Could you check a few things on this model? Use its own coordinates, in mm. Face numbers are marked on the shaded views. A direction names the side the tool comes from. Round coordinates to 2 decimals unless told otherwise and drop trailing zeros. Loops run counter-clockwise (first coordinate to the right, second up) from the corner with the lowest first, then second, coordinate; pieces in that order, holes last. Notation, with made-up numbers: M 61.25,79.5 L 75.25,79.5 A20 ccw 75.25,103.5 Z; hole C -5.5,84.5 d2. An arc over 180 degrees is marked long. Answer in a Markdown table with one row per item.
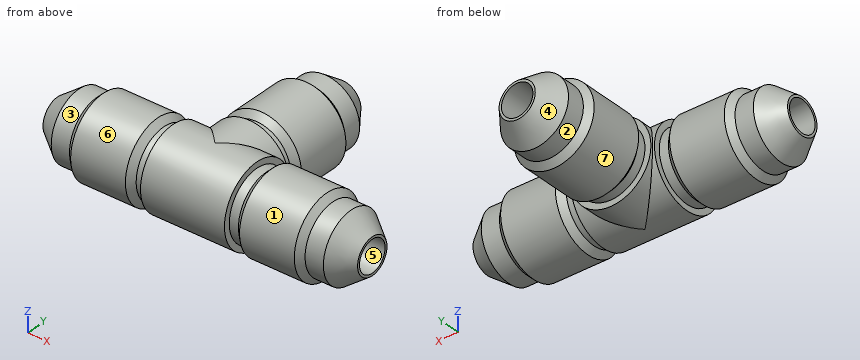
```python
from build123d import *

# Parameters (mm, degrees)
SKETCH2_R           = 5.55625
EXTRUDE1_DEPTH      = 16.002
SKETCH15_R          = 5.55625
BOSS_EXTRUDE1_DEPTH = 5.826125
SKETCH16_R          = 2.1844
CUT_EXTRUDE1_DEPTH  = 24.199372171
CIRPATTERN1_COUNT   = 3
CIRPATTERN1_ANGLE   = 180
SKETCH17_R          = 2.1844
CUT_EXTRUDE2_DEPTH  = 50.124404517
CUT_EXTRUDE3_REACH  = 37.458
SKETCH18_R          = 2.1844


with BuildPart() as part:
    # Sketch2 → Extrude1 (new body)
    with BuildSketch(Plane(origin=(-21.828125, 0, 0), x_dir=(0, 0, -1), z_dir=(1, 0, 0))):
        Circle(SKETCH2_R)
    extrude(amount=EXTRUDE1_DEPTH)

    # Sketch5 → Cut-Revolve1 (revolve, cut)
    with BuildSketch(Plane.XY, mode=Mode.PRIVATE) as cut_revolve1_sk:
        Polygon((-18.883013362, 4.731360803), (-16.343013362, 4.731360803), (-15.518124165, 5.55625), (-21.828125, 5.55625), (-21.828125, 2.51206), align=None)
        Polygon((-5.826125, 4.731360803), (-7.096125, 4.731360803), (-7.921014197, 5.55625), (-5.826125, 5.55625), align=None)
    revolve(cut_revolve1_sk.sketch.rotate(Axis((0, 0, 0), (-1, 0, 0)), 90), axis=Axis((0, 0, 0), (-1, 0, 0)), mode=Mode.SUBTRACT)

    # Sketch15 → Boss-Extrude1 (add)
    with BuildSketch(Plane(origin=(-5.826125, 0, 0), x_dir=(0, 0, -1), z_dir=(1, 0, 0))):
        Circle(SKETCH15_R)
    extrude(amount=BOSS_EXTRUDE1_DEPTH)

    # Sketch16 → Cut-Extrude1 (cut, through all)
    with BuildSketch(Plane(origin=(0, 0, 0), x_dir=(0, 0, -1), z_dir=(1, 0, 0))):
        Circle(SKETCH16_R)
    extrude(amount=-CUT_EXTRUDE1_DEPTH, mode=Mode.SUBTRACT)


with BuildPart() as cirpattern1_1:
    # CirPattern1: pattern copy
    add(part.part.rotate(Axis((0, 0, 0), (0, 0, -1)), 1 * CIRPATTERN1_ANGLE / (CIRPATTERN1_COUNT - 1)))

    # Sketch17 → Cut-Extrude2 (cut, through all)
    with BuildSketch(Plane.ZY.offset(21.828125)):
        with Locations(Location((0, 0, 0), (0, 0, 180))):
            Circle(SKETCH17_R)
    extrude(amount=-CUT_EXTRUDE2_DEPTH, mode=Mode.SUBTRACT)


with BuildPart() as cirpattern1_2:
    # CirPattern1: pattern copy
    add(part.part.rotate(Axis((0, 0, 0), (0, 0, -1)), 2 * CIRPATTERN1_ANGLE / (CIRPATTERN1_COUNT - 1)))


with BuildPart() as cirpattern1_1_1:
    add(cirpattern1_1.part)

    # Combine1: union part, CirPattern1_2
    add(part.part)
    add(cirpattern1_2.part)

    # Sketch18 → Cut-Extrude3 (cut, up to next)
    with BuildSketch(Plane(origin=(0, 21.828125, 0), x_dir=(1, 0, 0), z_dir=(0, 1, 0)), mode=Mode.PRIVATE) as cut_extrude3_sk1:
        with Locations(Location((0, 0, 0), (0, 0, 90))):
            Circle(SKETCH18_R)
    cut_extrude3_tool1 = extrude(cut_extrude3_sk1.sketch, amount=-CUT_EXTRUDE3_REACH, mode=Mode.PRIVATE) & cirpattern1_1_1.part
    add(cut_extrude3_tool1.solids().sort_by_distance((0, 21.828125, 0))[0], mode=Mode.SUBTRACT)


solid = cirpattern1_1_1.part
```
1) I want a section at B-B, the plane x = 0. Please give me the cut outline in (y, z), plus the area to 3 significant figures.
Computed:
| item | result |
|---|---|
| outline | M 0,-5.56 L 5.83,-5.56 L 5.83,-4.73 L 7.1,-4.73 L 7.92,-5.56 L 15.52,-5.56 L 16.34,-4.73 L 18.88,-4.73 L 21.83,-2.51 L 21.83,-2.18 L 0,-2.18 A2.18 cw 0,2.18 L 21.83,2.18 L 21.83,2.51 L 18.88,4.73 L 16.34,4.73 L 15.52,5.56 L 7.92,5.56 L 7.1,4.73 L 5.83,4.73 L 5.83,5.56 L 0,5.56 A5.56 ccw Z |
| area | 169 mm² |
2) I want a section at C-C, the plane z = 0. State how many separate pieces and enclosed holes the cut face has, plus the area to 3 significant figures.
Computed:
| item | result |
|---|---|
| separate pieces | 3 |
| enclosed holes | 0 |
| area | 332 mm² |
3) I need wall thicknesses on line 1 (X direction, y = 13.75, z = 0); line 2 (X direction, y = 17.5, z = 0); line 3 (Y direction, x = 0.5, z = 0). Which ranges of each line are inside material? Lowest first, please.
Computed:
| item | result |
|---|---|
| line 1 | x = -5.56 to -2.18, 2.18 to 5.56 |
| line 2 | x = -4.73 to -2.18, 2.18 to 4.73 |
| line 3 | y = -5.56 to -2.18 |
4) Will these pins go through, and if not, where does the flat tip stop? P1, Ø1.5, axis at x = -12, y = 5.5, coming from the -Z side; P2, Ø1, axis at x = -5, y = 10, coming from the -Z side; P3, Ø1, axis at x = -2, z = -4, coming from the +Y side.
Computed:
| item | result |
|---|---|
| P1 | stops at z = -2.88 |
| P2 | stops at z = -3.26 |
| P3 | stops at y = 19.89 |
5) If we mould it in two halves opening along Y, with no side actions, what happens to the marked faces 4, 5, 6 and 7? For each: released by +Y, released by -Y, zero draft, split by the parting line, or undercut.
Computed:
| item | result |
|---|---|
| face 4 | released by +Y |
| face 5 | undercut |
| face 6 | split by the parting line |
| face 7 | zero draft |
6) I want a section at D-D, the plane x = 6.5. Please give me the cut outline in (y, z), plus the area to 3 significant figures.
Computed:
| item | result |
|---|---|
| outline | C 0,0 d9.46; hole C 0,0 d4.37 |
| area | 55.3 mm² |
7) I want a section at A-A, the plane y = 11. Please give me the cut outline in (x, z).
Computed:
| item | result |
|---|---|
| outline | C 0,0 d11.11; hole C 0,0 d4.37 |
8) Which directions (+Z, -Z, +X, -X, +Y, -Y) give clear straight access to the entire face, cutting with the end or side of a thin tool? Please do the marked faces 1, 2 and 3.
Computed:
| item | result |
|---|---|
| face 1 | +X |
| face 2 | +Y |
| face 3 | -X |
